Input: part model. Units: mm. Frame: model coordinates. A direction names the side the tool comes from. Give positions to 0.01 mm unless a question says otherwise; leave off trailing zeros. Loops run counter-clockwise (first coordinate to the right, second up) from the corner with the lowest first, then second, coordinate; pieces in that order, holes last. Notation, with made-up numbers: (15, 78) -> (73, 78) arc R26 ccw to (73, 100) -> close; hole circle Ø10 at (-26.5, 26). An arc over 180 degrees is marked (long way). Use CSV: the item, a comma, the result in double quotes.
```python
from build123d import *

# Parameters (mm, degrees)
SKETCH1_R           = 100
BOSS_EXTRUDE1_DEPTH = 25
SKETCH2_R           = 15
BOSS_EXTRUDE2_DEPTH = 80
SKETCH3_R           = 10
CUT_EXTRUDE1_DEPTH  = 5


with BuildPart() as part:
    # Sketch1 → Boss-Extrude1 (new body)
    with BuildSketch(Plane.XY):
        Circle(SKETCH1_R)
    extrude(amount=BOSS_EXTRUDE1_DEPTH)

    # Sketch2 → Boss-Extrude2 (add)
    with BuildSketch(Plane.XY.offset(25)):
        Circle(SKETCH2_R)
    extrude(amount=BOSS_EXTRUDE2_DEPTH)

    # Sketch3 → Cut-Extrude1 (cut)
    with BuildSketch(Plane(origin=(0, 0, 0), x_dir=(-1, 0, 0), z_dir=(0, 0, -1))):
        with Locations((0, 50)):
            Circle(SKETCH3_R)
    extrude(amount=-CUT_EXTRUDE1_DEPTH, mode=Mode.SUBTRACT)


solid = part.part
```
1) Reachability of faces 4 (the flat face through (0, 0, 105)), 5 (the cylindrical face through (2.17, 40.24, 2.46)) from +Z, -Z, +X, -X, +Y, -Y: full face, straight path, thin tool, end or side. Return the list, or none.
From the geometry:
face 4,"+Z, +X, -X, +Y, -Y"
face 5,"-Z"
2) Section query D-D (y = 50). Return loops of the section in (x, z), then the cut area to 3 significant figures.
From the geometry:
outline,"(-86.6, 0) -> (-10, 0) -> (-10, 5) -> (10, 5) -> (10, 0) -> (86.6, 0) -> (86.6, 25) -> (-86.6, 25) -> close"
area,"4,230 mm^2"
3) Section query C-C (z = 51). Return loops of the section in (x, y), then the cut area to 3 significant figures.
From the geometry:
outline,"circle Ø30 at (0, 0)"
area,"707 mm^2"
4) Section query B-B (y = 0). Return loops of the section in (x, z).
From the geometry:
outline,"(-100, 0) -> (100, 0) -> (100, 25) -> (15, 25) -> (15, 105) -> (-15, 105) -> (-15, 25) -> (-100, 25) -> close"
5) Ray query, line 1 (Y direction, x = 0, z = 3.75); line 2 (Z direction, x = -62, y = 74.5); line 3 (Y direction, x = -31.5, z = 11.5). Return the intervals inside material, ascending.
From the geometry:
line 1,"y = -100 to 40, 60 to 100"
line 2,"z = 0 to 25"
line 3,"y = -94.91 to 94.91"
6) Contact query for flat-ended pins moving along their axis: pin 1 (12 mm diameter, centred on y = -14, z = 50.5, fed in from -X); pin 2 (12 mm diameter, centred on x = 17.5, z = 69.5, fed in from +Y); pin 3 (1.5 mm diameter, centred on y = 13.5, z = 80.5, fed in from -X). Output: stop coordinate, or through.
From the geometry:
pin 1,"stops at x = -12.69"
pin 2,"stops at y = 9.63"
pin 3,"stops at x = -7.9"
7) Section query A-A (x = 0). Return loops of the section in (y, z), then the cut area to 3 significant figures.
From the geometry:
outline,"(-100, 0) -> (40, 0) -> (40, 5) -> (60, 5) -> (60, 0) -> (100, 0) -> (100, 25) -> (15, 25) -> (15, 105) -> (-15, 105) -> (-15, 25) -> (-100, 25) -> close"
area,"7,300 mm^2"
8) Mould query, pull axis Y, two halves, no side actions, for faces 1 (the flat face through (-1, 1, 0)), 2 (the cylindrical face through (-14.985, 0.66, 64.44)), 3 (the flat face through (0, 50, 5)). Classes: pulls with the +Y half, pulls with the -Y half, needs draft (parallel to the pull), parting line crosses it, or undercut.
From the geometry:
face 1,"needs draft"
face 2,"parting line crosses it"
face 3,"undercut"
